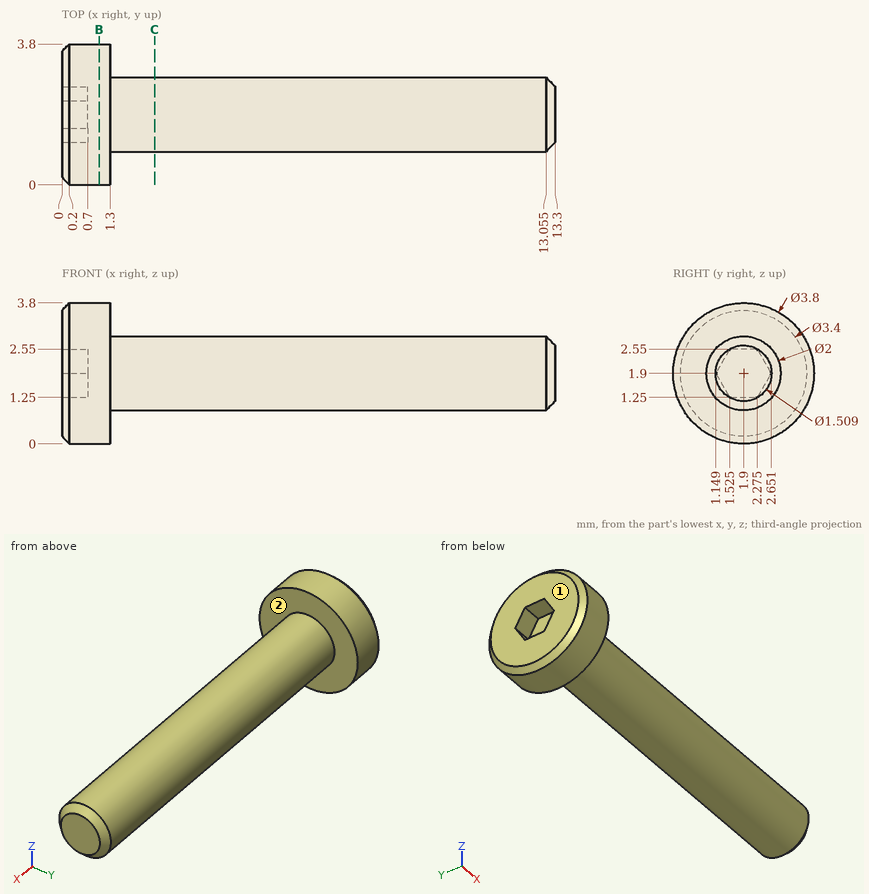
Could you check a few things on this drawing? It's one solid part, dimensions in mm from its lowest x, y, z. A direction names the side the tool comes from. Round coordinates to 2 decimals unless told otherwise and drop trailing zeros. Loops run counter-clockwise (first coordinate to the right, second up) from the corner with the lowest first, then second, coordinate; pieces in that order, holes last. Notation, with made-up numbers: (45.25, 58) -> (54.25, 58) arc R22 ccw to (54.25, 65) -> close; hole circle Ø8 at (33, 74). An arc over 180 degrees is marked (long way). Answer as CSV lines item,"result".
1. If we section it at C-C on x = 2.5: Please give me the cut outline in (y, z).
Final values:
outline,"circle Ø2 at (1.9, 1.9)"
2. If we section it at B-B on x = 1: Please give me the cut outline in (y, z).
Final values:
outline,"circle Ø3.8 at (1.9, 1.9)"
3. Which directions (+Z, -Z, +X, -X, +Y, -Y) give clear straight access to the entire face, cutting with the end or side of a thin tool? Please do the marked faces 1 and 2.
Final values:
face 1,"+Z, -Z, -X, +Y, -Y"
face 2,"+X"
4. For pin 1 (1 mm diameter, centred on x = 11.5, z = 2, fed in from -Y); pin 2 (1 mm diameter, centred on x = 3, y = 2, fed in from +Z), each with a flat end and sliding along its axis, tell me the tip position at first contact or that it passes through.
Final values:
pin 1,"stops at y = 0.9"
pin 2,"stops at z = 2.9"
5. If I drill on L1, parallel to X at y = 0.95, z = 2.55; L2, parallel to X at y = 1.6, z = 1.9; L3, parallel to Y at x = 7.75, z = 1.6 (1 decimal), over which ranges is the centre line in solid material (lowest first)?
Final values:
L1,"x = 0 to 1.3"
L2,"x = 0.7 to 13.3"
L3,"y = 0.9 to 2.9"
